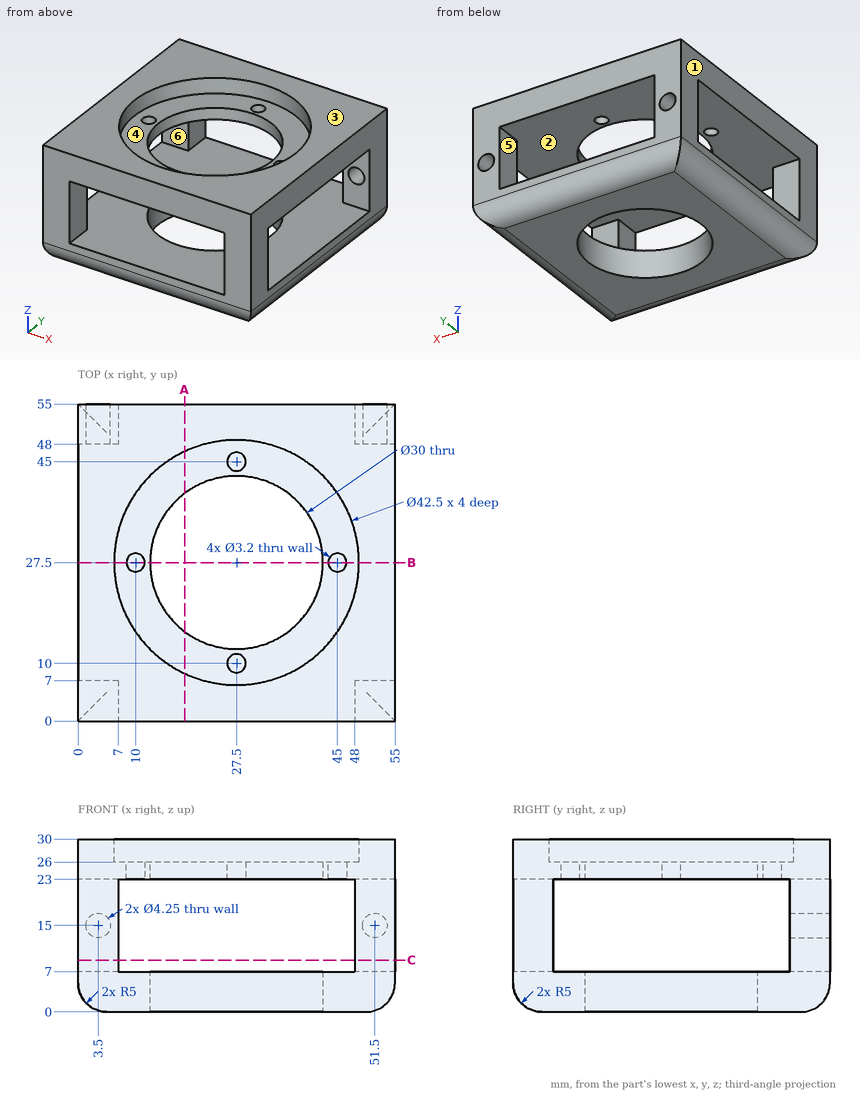
For this review, use the dimensioned drawing (mm, ordinates from the lowest corner) and the shaded views. A direction names the side the tool comes from. Coordinates: 2 decimals unless noted, no trailing zeros. Loops run counter-clockwise (first coordinate to the right, second up) from the corner with the lowest first, then second, coordinate; pieces in that order, holes last. Notation, with made-up numbers: (-7, -16.5) - (49, -16.5) arc R29 ccw to (49, 17.5) - close; hole circle Ø8 at (42, -27.75). An arc over 180 degrees is marked (long way). Use CSV: the item, a comma, the result in double quotes. Start each with the question number.
1) For pin 1 Ø21 at (x, y) = (31.5, 23) entering from +Z, flat-tipped, find the tip position at first contact; note if it passes through.
2) Tool access review of the marked faces 4, 5 and 6: name each direction out of +Z, -Z, +X, -X, +Y, -Y from which nothing blocks a thin tool from reaching the whole face with its end or side.
3) The part is to be moulded in two halves that separate along X. For the marked faces 1, 2 and 3, say which applies: +X half, -X half, draft (parallel to the pull), parting line (faces both ways), or undercut.
4) Consider section A-A on x = 18.5. Write out the cut boundary in (y, z).
5) Wall thickness on L1, parallel to Y at x = 27.5, z = 23.7; L2, parallel to Y at x = 27.5, z = 4.75; L3, parallel to Z at x = 39.5, y = 49: over which ranges is each line inside the solid? List them lowest first. Write a range as from..to.
6) Consider section B-B on y = 27.5. Give the number of separate pieces and of enclosed holes in the cut face, then the cut area to 3 significant figures.
7) Consider section C-C on z = 9. Write out the cut boundary in (x, y), then the cut area to 3 significant figures.
Geometry says:
1,pin 1,"z = 26"
2,face 4,"+Z"
2,face 5,"+Y, -Y"
2,face 6,"+X, -X"
3,face 1,"-X half"
3,face 2,"undercut"
3,face 3,"draft"
4,outline,"(0, 5) arc R5 ccw to (5, 0) - (15.5, 0) - (15.5, 7) - (0, 7) - close; (0, 23) - (15.5, 23) - (15.5, 26) - (8.25, 26) - (8.25, 30) - (0, 30) - close; (39.5, 0) - (50, 0) arc R5 ccw to (55, 5) - (55, 7) - (39.5, 7) - close; (39.5, 23) - (55, 23) - (55, 30) - (46.75, 30) - (46.75, 26) - (39.5, 26) - close"
5,L1,"0..8.4, 11.6..12.5, 42.5..43.4, 46.6..55"
5,L2,"0.01..12.5, 42.5..54.99"
5,L3,"0..7, 23..30"
6,separate pieces,"6"
6,enclosed holes,"0"
6,area,"270 mm^2"
7,outline,"(0, 0) - (7, 0) - (7, 7) - (0, 7) - close; (0, 48) - (7, 48) - (7, 55) - (0, 55) - close; (48, 0) - (55, 0) - (55, 7) - (48, 7) - close; (48, 48) - (55, 48) - (55, 55) - (48, 55) - close"
7,area,"196 mm^2"
